Here's how the part is built. I have some questions about the finished solid (model axes, mm). A direction names the side the tool comes from. Give positions to 0.01 mm unless a question says otherwise; leave off trailing zeros. Write each loop counter-clockwise with the first axis right and the second up, starting at its lowest first coordinate (ties: lowest second). Pieces come first, ordered by that corner, then holes. Notation, with made-up numbers: (-19.5, 74) -> (-12.5, 74) arc R32 ccw to (-12.5, 111) -> close; hole circle Ø6 at (30, 11.5). An arc over 180 degrees is marked (long way). Use one line per item in the form item = value.
Autodesk Inventor part; units mm, degrees
ref_plane "YZ Plane" through (0, 0, 0) normal (1, 0, 0) x (0, 1, 0)
ref_plane "XZ Plane" through (0, 0, 0) normal (0, 1, 0) x (-1, 0, 0)
ref_plane "XY Plane" through (0, 0, 0) normal (0, 0, 1) x (1, 0, 0)
sketch "Sketch1" plane through (0, 0, 0) normal (0, 0, 1) x (1, 0, 0)
  circle A0 centre (0, 0) radius 15.24
  circle A1 centre (0, 0) radius 25.4
  dimension "d0" = 30.48
  dimension "d1" = 50.8
extrude "Extrusion1" add sketch "Sketch1" along normal mid plane 40.64
sketch "Sketch2" plane through (0, 0, 0) normal (1, 0, 0) x (0, 1, 0)
  line L0 (25.4, -20.32) -> (15.24, -20.32)
  line L1 (15.24, -20.32) -> (15.24, 20.32)
  line L2 (15.24, 20.32) -> (25.4, 20.32)
  line L3 (25.4, 20.32) -> (25.4, -20.32)
  line L4 (-15.24, -20.32) -> (-25.4, -20.32)
  line L5 (-25.4, -20.32) -> (-25.4, 20.32)
  line L6 (-25.4, 20.32) -> (-15.24, 20.32)
  line L7 (-15.24, 20.32) -> (-15.24, -20.32)
  line L8 (25.4, -20.32) -> (15.24, -20.32)
  line L9 (15.24, -20.32) -> (15.24, 20.32)
  line L10 (15.24, 20.32) -> (25.4, 20.32)
  line L11 (25.4, 20.32) -> (25.4, -20.32)
  line L12 (-15.24, -20.32) -> (-25.4, -20.32)
  line L13 (-25.4, -20.32) -> (-25.4, 20.32)
  line L14 (-25.4, 20.32) -> (-15.24, 20.32)
  line L15 (-15.24, 20.32) -> (-15.24, -20.32)
  line L16 (-25.4, -20.32) -> (25.4, -20.32)
  line L17 (25.4, 20.32) -> (-25.4, 20.32)
  line L18 (-25.4, -20.32) -> (-53.34, -20.32)
  line L19 (-53.34, -20.32) -> (-53.34, -12.7)
  line L20 (-53.34, -12.7) -> (-25.4, -12.7)
  line L21 (-25.4, -12.7) -> (-25.4, -20.32)
  line L22 (25.4, 20.32) -> (-25.4, 20.32)
  line L23 (-25.4, 20.32) -> (-53.34, 20.32)
  line L24 (-53.34, 20.32) -> (-53.34, 12.7)
  line L25 (-53.34, 12.7) -> (-25.4, 12.7)
  line L26 (-25.4, 12.7) -> (-25.4, 20.32)
  line L27 (0, -28.448) -> (0, 28.448)
  point P0 (0, 0)
  dimension "d4" = 27.94
  dimension "d5" = 7.62
  dimension "d6" = 27.94
  dimension "d7" = 7.62
revolve "Revolution1" add sketch "Sketch2" angle 360 about axis through (0, 0, -10) along (0, 0, 1) contours L18 L19 L20 L5 | L5 L25 L24 L23
chamfer "Chamfer1" distance 1.27 angle 45 1 edges at (0, 53.34, -20.32) measured on face at (-31.6257, -42.9531, -15.24)
chamfer "Chamfer2" distance 1.27 angle 45 1 edges at (0, 53.34, -12.7) measured on face at (-31.6257, -42.9531, -14.8167)
chamfer "Chamfer3" distance 1.27 angle 45 2 edges at (0, 53.34, 20.32) (0, 53.34, 12.7) measured on face at (-31.6257, -42.9531, 17.78)
sketch "Sketch3" plane through (0, 0, 20.32) normal (0, 0, 1) x (1, 0, 0)
  circle A0 centre (0, 0) radius 40.64 construction
  circle A1 centre (0, 40.64) radius 6.35
  circle A2 centre (-35.1953, 20.32) radius 6.35
  circle A3 centre (-35.1953, -20.32) radius 6.35
  circle A4 centre (0, -40.64) radius 6.35
  circle A5 centre (35.1953, -20.32) radius 6.35
  circle A6 centre (35.1953, 20.32) radius 6.35
  dimension "d18" = 81.28
  dimension "d19" = 12.7
  dimension "d22" = 360
extrude "Extrusion2" cut sketch "Sketch3" against normal through all
equation "\"BendRadius\" = Thickness"
equation "\"BendReliefWidth\" = Thickness"
equation "\"BendReliefDepth\" = 0.5 * Thickness"
equation "\"CornerReliefSize\" = 4 * Thickness"
equation "\"MinimumRemnant\" = 2 * Thickness"
equation "\"TransitionRadius\" = BendRadius"
equation "\"JacobiRadiusSize\" = BendRadius"
equation "\"GapSize\" = Thickness"
properties part number "connecting rod hub" material "Brass, Soft Yellow"
Q1. I want a section at A-A, the plane y = 0. Write out the boundary of the cut face in (x, z), and give its area (3 significant figures).
Result set:
outline = (-53.34, -19.05) -> (-52.07, -20.32) -> (-15.24, -20.32) -> (-15.24, 20.32) -> (-52.07, 20.32) -> (-53.34, 19.05) -> (-53.34, 13.97) -> (-52.07, 12.7) -> (-25.4, 12.7) -> (-25.4, -12.7) -> (-52.07, -12.7) -> (-53.34, -13.97) -> close; (15.24, -20.32) -> (52.07, -20.32) -> (53.34, -19.05) -> (53.34, -13.97) -> (52.07, -12.7) -> (25.4, -12.7) -> (25.4, 12.7) -> (52.07, 12.7) -> (53.34, 13.97) -> (53.34, 19.05) -> (52.07, 20.32) -> (15.24, 20.32) -> close
area = 1,670 mm2
Q2. Which directions (+Z, -Z, +X, -X, +Y, -Y) give clear straight access to the entire face, cutting with the end or side of a thin tool? Please do faces 5 (the face through (-22.4, 12.3, -12.7)), 6 (the face through (-3.3, 14.88, -0.28)).
Result set:
face_5 = none
face_6 = +Z, -Z
Q3. Will these pins go through, and if not, where does the flat tip stop? pin 1 Ø3 at (y, z) = (18.5, -15.5) entering from +X; pin 2 Ø3 at (x, z) = (-34, 15) entering from -Y; pin 3 Ø1 at (x, z) = (-23, 6.5) entering from -Y.
Result set:
pin_1 = 50.56
pin_2 = -42.3
pin_3 = -11.79
Q4. If we mould it in two halves opening along X, with no side actions, what happens to faces 1 (the face through (-11, -11, 20.32)), 2 (the face through (-29.33, -22.75, 16.56)), 3 (the face through (41.25, 22.23, 16.56)), 4 (the face through (-52.886, 6.944, 16.474))? For each: +X half, -X half, draft (parallel to the pull), parting line (faces both ways), or undercut.
Result set:
face_1 = draft
face_2 = undercut
face_3 = undercut
face_4 = parting line
Q5. I want a section at B-B, the plane z = 11. Write out the boundary of the cut face in (x, y), and give its area (3 significant figures).
Result set:
outline = circle Ø50.8 at (0, 0); hole circle Ø30.48 at (0, 0)
area = 1,300 mm2
Q6. I want a section at C-C, the plane x = 0. Count the separate pieces of the cut face and the enclosed holes in it, and give its area (3 significant figures).
Result set:
separate_pieces = 6
enclosed_holes = 0
area = 1,280 mm2
Q7. If I drill on line 1 along Z through (x, y) = (32, 6); line 2 along X through (y, z) = (20, -14); line 3 along Y through (x, z) = (0, 0), over which ranges is the centre line in solid material (lowest first)? Write a range as from..to.
Result set:
line_1 = -20.32..-12.7, 12.7..20.32
line_2 = -49.45..-41.54, -28.85..28.85, 41.54..49.45
line_3 = -25.4..-15.24, 15.24..25.4
